Can you work these out from the model? Positions are in its coordinate system, mm. A direction names the side the tool comes from. Round coordinates to 2 decimals unless told otherwise and drop trailing zeros. Write each loop counter-clockwise with the first axis right and the second up, starting at its lowest first coordinate (ties: lowest second). Pieces come first, ordered by that corner, then holes. Notation, with made-up numbers: (-37.75, 32.5) -> (-11.75, 32.5) arc R12 cw to (-11.75, 52.5) -> close; hole circle Ø5 at (34.5, 50.25). An arc over 180 degrees is marked (long way). Write item = value, one per line. Start each with the question number.
1) Imagine slicing it at D-D, the plane z = 13.5. Please give me the cut outline in (x, y), then the cut area to 3 significant figures.
2) For faces 4 (the face through (-3.8, 6.3, -3.8)), 5 (the face through (0, 17, -5.6)), 6 (the face through (0, 0, -16)), which set-ups out of +Z, -Z, +X, -X, +Y, -Y let a thin tool reach every point of the face, with its end or its side?
3) If I drill on line 1 (Y direction, x = 15.5, z = -3); line 2 (Z direction, x = -0.5, y = 5) (3 decimals); line 3 (Z direction, x = 3, y = 13), over which ranges is the centre line in solid material (lowest first)?
4) Imagine slicing it at B-B, the plane z = -18.5. Please give me the cut outline in (x, y).
5) Imagine slicing it at C-C, the plane z = 4. Please give me the cut outline in (x, y).
6) I'm going to push flat-ended pins straight in: pin 1 (12 mm diameter, centred on x = -12.5, y = 6, fed in from +Z) (3 decimals); pin 2 (12 mm diameter, centred on y = 14.5, z = 3.5, fed in from +X); pin 3 (1.9 mm diameter, centred on x = 1.5, y = 16.5, fed in from +Z). Where does each tip first touch, or does it pass through?
7) Thinking about a two-plate mould opening in Z: for faces 1 (the face through (4.872, 16.925, -2.761)), 2 (the face through (-4.336, 24.284, 19.524)), 3 (the face through (-3, 9, -9.975)), which applies, +Z half, -Z half, draft (parallel to the pull), parting line (faces both ways), or undercut?
from build123d import *

# Parameters (mm, degrees)
BOSS_EXTRUDE1_DEPTH      = 12.7
SKETCH2_R                = 3.445005279
BOSS_EXTRUDE2_DEPTH      = 4.6
BOSS_EXTRUDE2_DEPTH_BACK = 2
BOSS_EXTRUDE3_DEPTH      = 11.3
SKETCH4_R                = 5.15
BOSS_EXTRUDE4_DEPTH      = 9
BOSS_EXTRUDE5_DEPTH      = 8.57
SKETCH6_R                = 2.5
BOSS_EXTRUDE6_DEPTH      = 6
BOSS_EXTRUDE7_START      = -2
SKETCH7_R                = 20
BOSS_EXTRUDE7_DEPTH      = 2


with BuildPart() as part:
    # Sketch1 → Boss-Extrude1 (new body)
    with BuildSketch(Plane(origin=(0, 0, 0), x_dir=(1, 0, 0), z_dir=(0, 1, 0))):
        Polygon((-2.226397898, -5.375), (2.226397898, -5.375), (5.375, -2.226397898), (5.375, 2.226397898), (2.226397898, 5.375), (-2.226397898, 5.375), (-5.375, 2.226397898), (-5.375, -2.226397898), align=None)
    extrude(amount=BOSS_EXTRUDE1_DEPTH)

    # Sketch2 → Boss-Extrude2 (add, two sides)
    with BuildSketch(Plane(origin=(0, 0, -5.375), x_dir=(-1, 0, 0), z_dir=(0, 0, -1))) as boss_extrude2_sk:
        with Locations((0, 6.35)):
            Circle(SKETCH2_R)
    extrude(amount=BOSS_EXTRUDE2_DEPTH)
    extrude(boss_extrude2_sk.sketch, amount=-BOSS_EXTRUDE2_DEPTH_BACK)

    # Sketch3 → Boss-Extrude3 (add)
    with BuildSketch(Plane(origin=(0, 0, -9.975), x_dir=(-1, 0, 0), z_dir=(0, 0, -1))):
        Polygon((7.332348419, 6.35), (3.666174209, 12.7), (-3.666174209, 12.7), (-7.332348419, 6.35), (-3.666174209, 0), (3.666174209, 0), align=None)
    extrude(amount=BOSS_EXTRUDE3_DEPTH)

    # Sketch4 → Boss-Extrude4 (add)
    with BuildSketch(Plane.XZ):
        Circle(SKETCH4_R)
    extrude(amount=BOSS_EXTRUDE4_DEPTH)

    # Sketch5 → Boss-Extrude5 (add)
    with BuildSketch(Plane(origin=(0, 12.7, 0), x_dir=(1, 0, 0), z_dir=(0, 1, 0))):
        Polygon((6.466323015, 0), (3.233161507, 5.6), (-3.233161507, 5.6), (-6.466323015, 0), (-3.233161507, -5.6), (3.233161507, -5.6), align=None)
    extrude(amount=BOSS_EXTRUDE5_DEPTH)

    # Sketch6 → Boss-Extrude6 (add)
    with BuildSketch(Plane(origin=(0, 21.27, 0), x_dir=(1, 0, 0), z_dir=(0, 1, 0))):
        Circle(SKETCH6_R)
    extrude(amount=BOSS_EXTRUDE6_DEPTH)

    # Sketch7 → Boss-Extrude7 (add)
    with BuildSketch(Plane(origin=(0, 27.27, 0), x_dir=(1, 0, 0), z_dir=(0, 1, 0)).offset(BOSS_EXTRUDE7_START)):
        Circle(SKETCH7_R)
    extrude(amount=-BOSS_EXTRUDE7_DEPTH)


solid = part.part
Reported:
q1.outline = (-14.76, 23.27) -> (14.76, 23.27) -> (14.76, 25.27) -> (-14.76, 25.27) -> close
q1.area = 59.0 mm²
q2.face_4 = -X
q2.face_5 = -Z, +X, -X
q2.face_6 = -Z, +X, -X, -Y
q3.line_1 = 23.27 to 25.27
q3.line_2 = -21.275 to 5.375
q3.line_3 = -5.6 to 5.6
q4.outline = (-7.6, 23.27) -> (7.6, 23.27) -> (7.6, 25.27) -> (-7.6, 25.27) -> close; (-7.33, 6.35) -> (-3.67, 0) -> (3.67, 0) -> (7.33, 6.35) -> (3.67, 12.7) -> (-3.67, 12.7) -> close
q5.outline = (-19.6, 23.27) -> (19.6, 23.27) -> (19.6, 25.27) -> (-19.6, 25.27) -> close; (-4.16, 12.7) -> (-3.6, 12.7) -> (-3.6, 0) -> (-3.24, 0) -> (-3.24, -9) -> (3.24, -9) -> (3.24, 0) -> (3.6, 0) -> (3.6, 12.7) -> (4.16, 12.7) -> (4.16, 21.27) -> (-4.16, 21.27) -> close
q6.pin_1 = -9.975
q6.pin_2 = 6.47
q6.pin_3 = 5.6
q7.face_1 = -Z half
q7.face_2 = parting line
q7.face_3 = undercut
